For this review, use the dimensioned drawing (mm, ordinates from the lowest corner) and the shaded views. A direction names the side the tool comes from. Round coordinates to 2 decimals unless told otherwise and drop trailing zeros. Loops run counter-clockwise (first coordinate to the right, second up) from the corner with the lowest first, then second, coordinate; pieces in that order, holes last. Notation, with made-up numbers: M 48,22.5 L 99,22.5 A13 ccw 99,33.5 Z; hole C 2.5,45.25 d9. An arc over 180 degrees is marked long. One line per item, written item: value. Start each with the question number.
Item 1: Mouldability with a two-part tool opening along X and no side actions: class the marked faces 4, 5 and 6 as released by +X, released by -X, zero draft, split by the parting line, or undercut.
Item 2: We need section D-D (z = 53.5). Write out the cut boundary in (x, y) (1 decimal), then the cut area to 3 significant figures.
Item 3: For line 1 along Y through (x, z) = (34.5, 72); line 2 along X through (y, z) = (8.5, 39.5) (1 decimal); line 3 along Z through (x, y) = (45.5, 6.5), list the stretches that pass through material, from the lowest coordinate up.
Item 4: We need section C-C (z = 22). Write out the cut boundary in (x, y).
Item 5: We need section B-B (x = 45.5). Write out the cut boundary in (y, z).
Item 6: For the marked faces 1, 2 and 3, list the 3-axis set-ups (+Z, -Z, +X, -X, +Y, -Y) from which the entire face can be reached by the end or side of a thin tool; tool diameter is ignored.
Item 7: Clearance check with flat-ended pins moving along their axes: pin 1 (10 mm diameter, centred on x = 50, y = 28.5, fed in from -Z); pin 2 (2 mm diameter, centred on y = 31.5, z = 10.5, fed in from -X) (1 decimal); pin 3 (12 mm diameter, centred on x = 16, y = 28.5, fed in from -Z) (1 decimal). State where each tip first meets the part, or that it passes through.
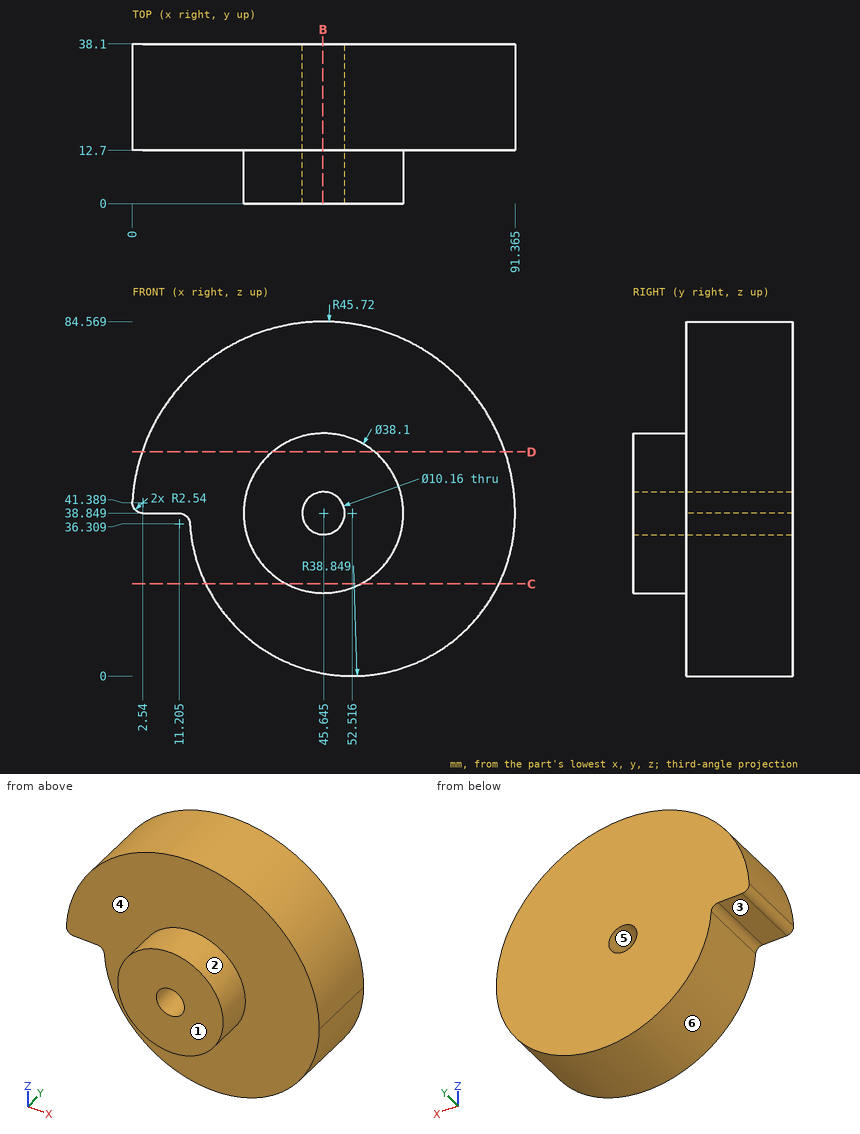
A:
1. face 4: zero draft
1. face 5: undercut
1. face 6: split by the parting line
2. outline: M 2.3,12.7 L 33.5,12.7 L 33.5,0 L 57.8,0 L 57.8,12.7 L 89,12.7 L 89,38.1 L 2.3,38.1 Z
2. area: 2,510 mm2
3. line 1: 12.7 to 38.1
3. line 2: 26.6 to 40.6, 50.7 to 64.7
3. line 3: 19.8 to 33.77, 43.93 to 57.9
4. outline: M 17.51,12.7 L 36.76,12.7 L 36.76,0 L 54.53,0 L 54.53,12.7 L 87.52,12.7 L 87.52,38.1 L 17.51,38.1 Z
5. outline: M 0,19.8 L 12.7,19.8 L 12.7,0.64 L 38.1,0.64 L 38.1,33.77 L 0,33.77 Z; M 0,43.93 L 38.1,43.93 L 38.1,84.57 L 12.7,84.57 L 12.7,57.9 L 0,57.9 Z
6. face 1: +Z, -Z, +X, -X, -Y
6. face 2: -Y
6. face 3: -Z, -X, +Y, -Y
7. pin 1: z = 0
7. pin 2: x = 24.9
7. pin 3: z = 14.8
